from build123d import *

# Parameters (mm, degrees)
SKETCH1_W                        = 76.2
SKETCH1_H                        = 9.525
SKETCH2_R                        = 50.8
BOSS_EXTRUDE1_DEPTH              = 12.7
SKETCH3_R                        = 12.7
BOSS_EXTRUDE2_DEPTH              = 50.8
F_3_8_0_375_DIAMETER_HOLE1_D     = 9.525
F_2_4_5_TAPPED_HOLE1_D           = 12.7
F_2_4_5_TAPPED_HOLE1_CBORE_D     = 50.8
F_2_4_5_TAPPED_HOLE1_CBORE_DEPTH = 3.175
F_7_0_201_DIAMETER_HOLE1_D       = 5.1054
F_7_0_201_DIAMETER_HOLE1_DEPTH   = 12.7
F_7_0_201_DIAMETER_HOLE1_TIP     = 1.533816902
CHAMFER1_SIZE                    = 0.622299999
CHAMFER1_SIZE2                   = 0.622300001


with BuildPart() as part:
    # Sketch1 → Revolve1 (revolve)
    with BuildSketch(Plane.XY, mode=Mode.PRIVATE) as revolve1_sk:
        with Locations((38.1, 4.7625)):
            Rectangle(SKETCH1_W, SKETCH1_H)
    revolve(revolve1_sk.sketch.rotate(Axis((0, 9.525, 0), (0, -1, 0)), 270), axis=Axis((0, 9.525, 0), (0, -1, 0)))

    # Sketch2 → Boss-Extrude1 (add)
    with BuildSketch(Plane(origin=(0, 9.525, 0), x_dir=(-1, 0, 0), z_dir=(0, 1, 0))):
        with Locations(Location((0, 0, 0), (0, 0, 90))):
            Circle(SKETCH2_R)
    extrude(amount=BOSS_EXTRUDE1_DEPTH)

    # Sketch3 → Boss-Extrude2 (add)
    with BuildSketch(Plane(origin=(0, 22.225, 0), x_dir=(-1, 0, 0), z_dir=(0, 1, 0))):
        with Locations(Location((0, 0, 0), (0, 0, 90))):
            Circle(SKETCH3_R)
    extrude(amount=BOSS_EXTRUDE2_DEPTH)

    # 3/8 (0.375) Diameter Hole1 (through all)
    with Locations(Plane(origin=(0, 9.525, 0), x_dir=(1, 0, 0), z_dir=(0, 1, 0))):
        with Locations((63.5, 0), (54.99261314, 31.75), (31.75, 54.99261314), (0, -63.5), (-31.75, -54.99261314), (-54.99261314, -31.75), (-63.5, 0), (-54.99261314, 31.75), (-31.75, 54.99261314), (0, 63.5), (31.75, -54.99261314), (54.99261314, -31.75)):
            Hole(F_3_8_0_375_DIAMETER_HOLE1_D / 2)

    # 2-4.5 Tapped Hole1 (through all)
    with Locations(Plane(origin=(0, 0, 0), x_dir=(-1, 0, 0), z_dir=(0, -1, 0))):
        with Locations((0, 0)):
            CounterBoreHole(F_2_4_5_TAPPED_HOLE1_D / 2, F_2_4_5_TAPPED_HOLE1_CBORE_D / 2, F_2_4_5_TAPPED_HOLE1_CBORE_DEPTH)

    # #7 (0.201) Diameter Hole1
    with Locations(Plane(origin=(0, 22.225, 0), x_dir=(1, 0, 0), z_dir=(0, 1, 0))):
        with Locations((31.75, 0), (0, -31.75), (0, 31.75), (-31.75, 0)):
            Hole(F_7_0_201_DIAMETER_HOLE1_D / 2, depth=F_7_0_201_DIAMETER_HOLE1_DEPTH)
            with Locations((0, 0, -(F_7_0_201_DIAMETER_HOLE1_DEPTH + F_7_0_201_DIAMETER_HOLE1_TIP / 2))):  # 118° drill point
                Cone(0, F_7_0_201_DIAMETER_HOLE1_D / 2, F_7_0_201_DIAMETER_HOLE1_TIP, mode=Mode.SUBTRACT)

    # Chamfer1
    chamfer1_edges = [part.edges().sort_by_distance(p)[0] for p in [
        (-29.1973, 22.225, 0),
        (2.5527, 22.225, -31.75),
        (2.5527, 22.225, 31.75),
        (34.3027, 22.225, 0),
    ]]
    chamfer1_side = [part.faces().sort_by_distance(p)[0] for p in [
        (0, 22.225, -49.363159021),
    ]]
    chamfer(chamfer1_edges, length=CHAMFER1_SIZE, length2=CHAMFER1_SIZE2, reference=chamfer1_side[0])


solid = part.part
Design review of the part built by this model. Coordinates are the model's own, in mm. A direction names the side the tool comes from. Give positions to 0.01 mm unless a question says otherwise; leave off trailing zeros. Loops run counter-clockwise (first coordinate to the right, second up) from the corner with the lowest first, then second, coordinate; pieces in that order, holes last. Notation, with made-up numbers: (63, 10) -> (73, 10) arc R11 ccw to (73, 25) -> close; hole circle Ø1 at (61.5, 64.5). An arc over 180 degrees is marked (long way). One line per question, with ' | ' between items. Start each with the question number.
(1) Draft analysis for pull direction X (two halves, no side actions). For faces 1 (the face through (-50, 9.525, 16)), 2 (the face through (5.506, 1.565, 24.796)), 3 (the face through (-7.7, 47.3, -10.1)), state which applies: +X half, -X half, draft (parallel to the pull), parting line (faces both ways), or undercut.
(2) We need section C-C (x = -44.5). State the section outline as (y, z) points (3 decimals).
(3) Insertion check: P1, Ø12.5, axis at x = 0, z = 63.5, coming from the +Y side (3 decimals); P2, Ø4, axis at x = 0, z = -31.75, coming from the +Y side; P3, Ø1, axis at y = 12, z = -0.5, coming from the +X side. Each pin has a flat end and moves straight along its axis. Give the tip position at first contact, or say it passes through.
(4) We need section D-D (y = 68). State the section outline as (x, z) points.
(5) For faces 4 (the face through (-5, 3.175, 5)), 5 (the face through (-36.29, 4.7, 53.56)), 6 (the face through (0.553, 15.479, 34.242)), list the 3-axis set-ups (+Z, -Z, +X, -X, +Y, -Y) from which the entire face can be reached by the end or side of a thin tool; tool diameter is ignored.
(6) We need section B-B (x = -63.5). State the section outline as (y, z) points (1 decimal).
(7) For line 1 (Z direction, x = -31, y = 2); line 2 (Y direction, x = -66, z = 26.5) (3 decimals); line 3 (X direction, y = 3.25, z = -63.5), list the stretches that pass through material, from the lowest coordinate up.
(8) We need section A-A (z = 63.5). State the section outline as (x, y) points (1 decimal).
The answers:
1) face 1: draft | face 2: undercut | face 3: parting line
2) outline: (0, -61.856) -> (9.525, -61.856) -> (9.525, -24.503) -> (22.225, -24.503) -> (22.225, 24.503) -> (9.525, 24.503) -> (9.525, 61.856) -> (0, 61.856) -> close
3) P1: stops at y = 9.525 | P2: stops at y = 9.19 | P3: stops at x = 50.8
4) outline: circle Ø25.4 at (0, 0); hole circle Ø12.7 at (0, 0)
5) face 4: -Y | face 5: +Y, -Y | face 6: +Y
6) outline: (0, -42.1) -> (9.5, -42.1) -> (9.5, -4.8) -> (0, -4.8) -> close; (0, 4.8) -> (9.5, 4.8) -> (9.5, 42.1) -> (0, 42.1) -> close
7) line 1: z = -69.61 to -59.7, -50.29 to 50.29, 59.7 to 69.61 | line 2: y = 0 to 9.525 | line 3: x = -42.12 to -4.76, 4.76 to 42.12
8) outline: (-42.1, 0) -> (-4.8, 0) -> (-4.8, 9.5) -> (-42.1, 9.5) -> close; (4.8, 0) -> (42.1, 0) -> (42.1, 9.5) -> (4.8, 9.5) -> close
